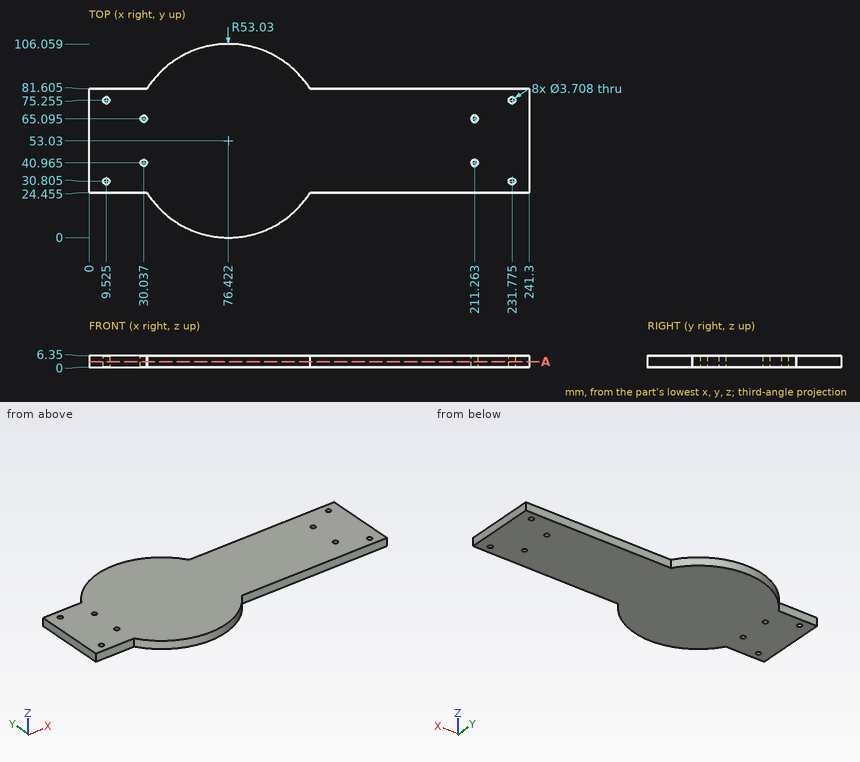
Check sheet for the drawn part. Datum: minimum x, y, z corner. Units: mm. Round coordinates to 2 decimals unless told otherwise and drop trailing zeros.
Item 1: Thickness scan on line 1 (Y direction, x = 213.5, z = 1) (1 decimal); line 2 (X direction, y = 63.5, z = 2.5) (1 decimal); line 3 (X direction, y = 64, z = 0.5) (1 decimal). Record the ranges inside material, lowest first.
Item 2: Gauge pin test, flat end, axial feed: pin 1 (1.9 mm diameter, centred on x = 11.5, z = 2.5, fed in from +Y) (1 decimal). Record the tip position at first contact, or that the pin passes through.
Item 3: Cross-section at A-A on z = 3. Count the separate pieces of the cut face and the enclosed holes in it, then the cut area to 3 significant figures.
Answer sheet:
1. line 1: y = 24.5 to 81.6
1. line 2: x = 0 to 29.1, 31 to 210.3, 212.2 to 241.3
1. line 3: x = 0 to 28.5, 31.5 to 209.8, 212.8 to 241.3
2. pin 1: stops at y = 81.6
3. separate pieces: 1
3. enclosed holes: 8
3. area: 16,800 mm2
